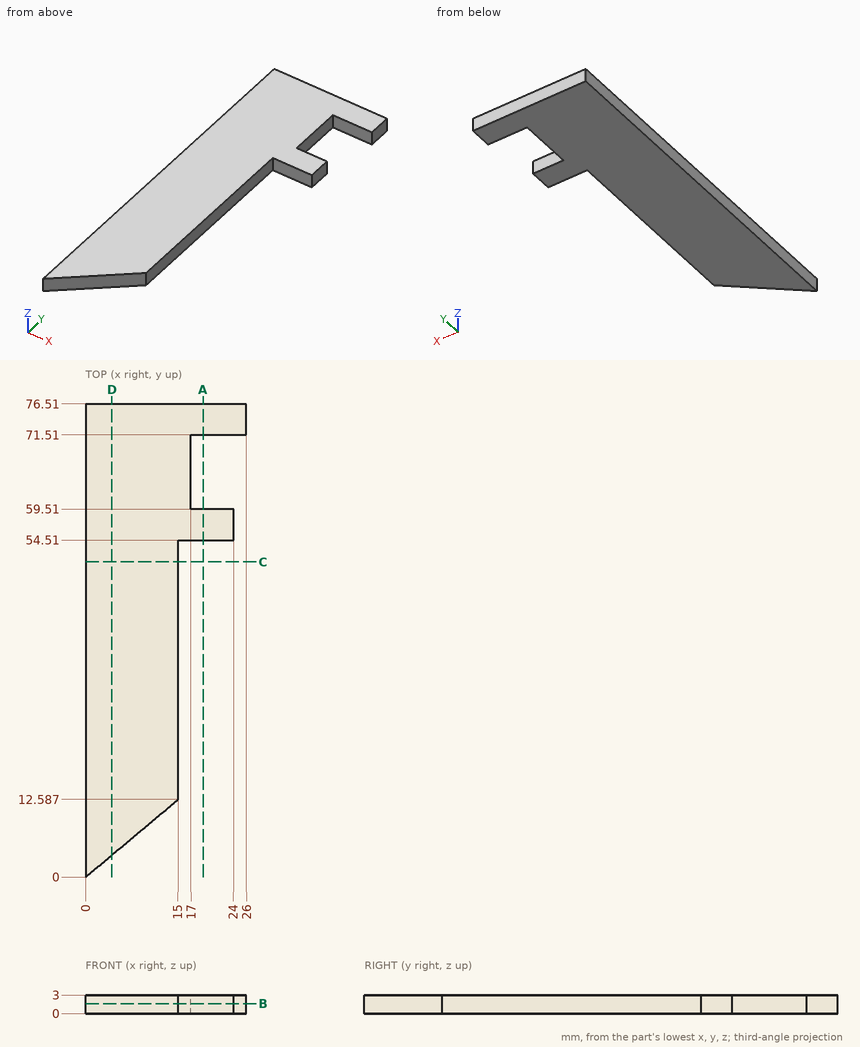
Verification items for this drawing (mm, ordinates from the low corner). Coordinates: 2 decimals unless noted, no trailing zeros. Order: outer loops, then holes, each group sorted by start corner. A loop starts at its lowest first (then second) coordinate and runs counter-clockwise, first axis right, second up. Notation, with made-up numbers: (43, 45) - (50, 45) arc R33 cw to (50, 78) - close; hole circle Ø4 at (-3.5, 44.5). An arc over 180 degrees is marked (long way). Answer in a Markdown table with one row per item. Add a question column.
1. Material ranges on L1, parallel to Y at x = 19.5, z = 1.5; L2, parallel to X at y = 57.5, z = 0.95; L3, parallel to X at y = 45, z = 0.9, recorded low to high. Write a range as [from, to].
2. Section check B-B (z = 1.65). Enter the section's corners in (x, y), plus the area to 3 significant figures.
3. Section check C-C (y = 51). Enter the section's corners in (x, z).
4. Gauge pin test, flat ends, axial feed: pin 1 Ø1.5 at (x, z) = (20, 1.5) entering from -Y; pin 2 Ø1.5 at (y, z) = (66, 1.5) entering from +X. Record the tip position at first contact, or that the pin passes through.
5. Section check D-D (x = 4.25). Enter the section's corners in (y, z).
6. Section check A-A (x = 19). Enter the section's corners in (y, z).
Data:
| question | item | result |
|---|---|---|
| 1 | L1 | y = [54.51, 59.51], [71.51, 76.51] |
| 1 | L2 | x = [0, 24] |
| 1 | L3 | x = [0, 15] |
| 2 | outline | (0, 0) - (15, 12.59) - (15, 54.51) - (24, 54.51) - (24, 59.51) - (17, 59.51) - (17, 71.51) - (26, 71.51) - (26, 76.51) - (0, 76.51) - close |
| 2 | area | 1,180 mm² |
| 3 | outline | (0, 0) - (15, 0) - (15, 3) - (0, 3) - close |
| 4 | pin 1 | stops at y = 54.51 |
| 4 | pin 2 | stops at x = 17 |
| 5 | outline | (3.57, 0) - (76.51, 0) - (76.51, 3) - (3.57, 3) - close |
| 6 | outline | (54.51, 0) - (59.51, 0) - (59.51, 3) - (54.51, 3) - close; (71.51, 0) - (76.51, 0) - (76.51, 3) - (71.51, 3) - close |
